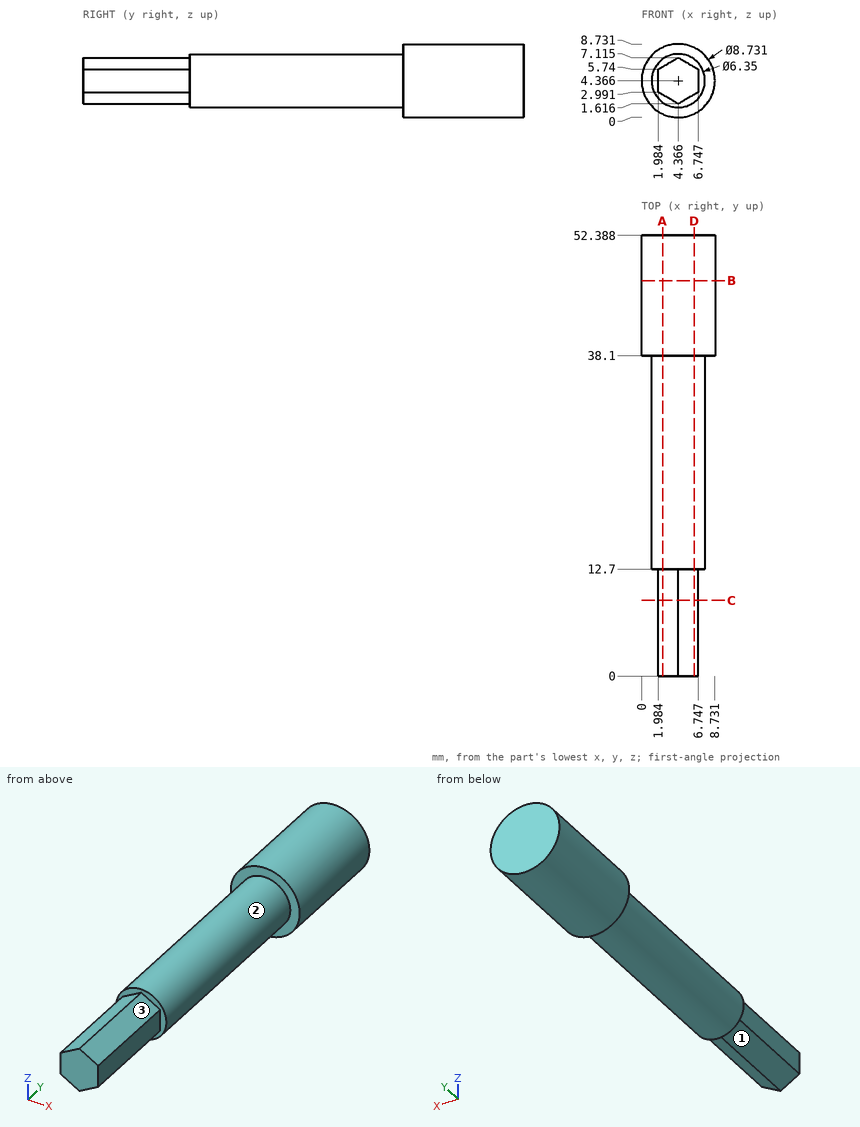
Could you check a few things on this drawing? It's one solid part, dimensions in mm from its lowest x, y, z. A direction names the side the tool comes from. Coordinates: 2 decimals unless noted, no trailing zeros. Write each loop counter-clockwise with the first axis right and the second up, starting at its lowest first coordinate (ties: lowest second). Pieces come first, ordered by that corner, then holes. Notation, with made-up numbers: M 3.5,26 L 51.5,26 A25 ccw 51.5,48 Z; hole C 64,71.25 d5. An arc over 180 degrees is marked long. Answer as CSV lines item,"result". Start each with the question number.
Q1. I need wall thicknesses on probe 1 along Z at (x, y) = (4.5, 13); probe 2 along Y at (x, z) = (7, 1.75); probe 3 along X at (y, z) = (38.5, 4.25). Which ranges of each line are inside material? Lowest first, please. Write a range as [from, to].
Q2. Suppose I cut it at D-D, the plane x = 6.25. List the corners of the cut face in (y, z) for me.
Q3. Suppose I cut it at C-C, the plane y = 9. List the corners of the cut face in (x, z) for me (1 decimal).
Q4. Suppose I cut it at A-A, the plane x = 2.5. List the corners of the cut face in (y, z) for me (1 decimal), then the cut area to 3 significant figures.
Q5. Suppose I cut it at B-B, the plane y = 47. List the corners of the cut face in (x, z) for me (1 decimal).
Q6. For the marked faces 1, 2 and 3, which set-ups out of +Z, -Z, +X, -X, +Y, -Y let a thin tool reach every point of the face, with its end or its side?
Q7. Will these pins go through, and if not, where does the flat tip stop? pin 1 Ø0.8 at (y, z) = (6, 4.5) entering from +X; pin 2 Ø3 at (y, z) = (3.5, 5) entering from -X; pin 3 Ø4 at (x, y) = (7, 35.5) entering from -Z (1 decimal).
Entries:
1,probe 1,"z = [1.19, 7.54]"
1,probe 2,"y = [38.1, 52.39]"
1,probe 3,"x = [0, 8.73]"
2,outline,"M 0,2.7 L 12.7,2.7 L 12.7,1.81 L 38.1,1.81 L 38.1,0.43 L 52.39,0.43 L 52.39,8.3 L 38.1,8.3 L 38.1,6.92 L 12.7,6.92 L 12.7,6.03 L 0,6.03 Z"
3,outline,"M 2,3 L 4.4,1.6 L 6.7,3 L 6.7,5.7 L 4.4,7.1 L 2,5.7 Z"
4,outline,"M 0,2.7 L 12.7,2.7 L 12.7,1.8 L 38.1,1.8 L 38.1,0.4 L 52.4,0.4 L 52.4,8.3 L 38.1,8.3 L 38.1,6.9 L 12.7,6.9 L 12.7,6 L 0,6 Z"
4,area,"286 mm²"
5,outline,"C 4.4,4.4 d8.7"
6,face 1,"-Z, -X, -Y"
6,face 2,"-Y"
6,face 3,"+Z, +X, -Y"
7,pin 1,"stops at x = 6.75"
7,pin 2,"stops at x = 1.98"
7,pin 3,"stops at z = 1.3"
